Part model, mm, in its own coordinate system. A direction names the side the tool comes from. Coordinates: 2 decimals unless noted, no trailing zeros. Order: outer loops, then holes, each group sorted by start corner. A loop starts at its lowest first (then second) coordinate and runs counter-clockwise, first axis right, second up. Notation, with made-up numbers: M 70.25,73.5 L 128.25,73.5 A24 ccw 128.25,91.5 Z; hole C 50,55.25 d8. An arc over 180 degrees is marked long. Write item = value, one per line. Start each with the question number.
from build123d import *

# Parameters (mm, degrees)
SKETCH1_W           = 10
SKETCH1_H           = 10
BOSS_EXTRUDE1_DEPTH = 10
SKETCH2_R           = 2.5
BOSS_EXTRUDE2_DEPTH = 10
SKETCH3_R           = 2.5
CUT_EXTRUDE1_DEPTH  = 10
SKETCH4_R           = 2.5
CUT_EXTRUDE2_DEPTH  = 10


with BuildPart() as part:
    # Sketch1 → Boss-Extrude1 (new body)
    with BuildSketch(Plane.XY):
        with Locations((5, 5)):
            Rectangle(SKETCH1_W, SKETCH1_H)
    extrude(amount=BOSS_EXTRUDE1_DEPTH)

    # Sketch2 → Boss-Extrude2 (add)
    with BuildSketch(Plane(origin=(0, 10, 0), x_dir=(1, 0, 0), z_dir=(0, 1, 0))):
        with Locations(Location((5, -5, 0), (0, 0, 270))):
            Circle(SKETCH2_R)
    extrude(amount=BOSS_EXTRUDE2_DEPTH)

    # Sketch3 → Cut-Extrude1 (cut)
    with BuildSketch(Plane.XY.offset(10)):
        with Locations((5, 5)):
            Circle(SKETCH3_R)
    extrude(amount=-CUT_EXTRUDE1_DEPTH, mode=Mode.SUBTRACT)

    # Sketch4 → Cut-Extrude2 (cut)
    with BuildSketch(Plane(origin=(10, 0, 0), x_dir=(0, 0, -1), z_dir=(1, 0, 0))):
        with Locations(Location((-5, 5, 0), (0, 0, 90))):
            Circle(SKETCH4_R)
    extrude(amount=-CUT_EXTRUDE2_DEPTH, mode=Mode.SUBTRACT)


solid = part.part
Item 1: Cut at C-C, the plane x = 7. Write the cut outline in (y, z), and give its area (3 significant figures).
Item 2: 3-axis set-ups, long thin cutter, end or side, ignore diameter. For faces 1 (the flat face through (3, 7, 0)), 2 (the cylindrical face through (5.751, 14.93, 7.385)): which of +Z, -Z, +X, -X, +Y, -Y reach the whole face in a straight line?
Item 3: Flat gauge pins, fed straight in: pin 1 (4 mm diameter, centred on x = 5, y = 5, fed in from -Z); pin 2 (4 mm diameter, centred on y = 15.5, z = 2, fed in from -X). Where does each tip first touch, or does it go through?
Item 4: Cut at D-D, the plane x = 8.25. Write the cut outline in (y, z), and give its area (3 significant figures).
Item 5: Wall check: line 1 along Y through (x, z) = (5, 8.25); line 2 along Y through (x, z) = (5, 6.25). Give the ranges that are in metal, low to high. Write a range as [from, to].
Item 6: Cut at B-B, the plane z = 3. Write the cut outline in (x, y), and give its area (3 significant figures).
Item 7: Pull direction Y, two halves, no side cores. Call faces 3 (the flat face through (3, 10, 3)), 4 (the cylindrical face through (6.34, 7.11, 8.09)), 5 (the flat face through (10, 3, 3)): pulls with the +Y half, pulls with the -Y half, needs draft (parallel to the pull), parting line crosses it, or undercut.
Item 8: Cut at A-A, the plane y = 5. Write the cut outline in (x, z), and give its area (3 significant figures).
Filled sheet:
q1.outline = M 0,0 L 3.5,0 L 3.5,3 A2.5 cw 3.5,7 L 3.5,10 L 0,10 Z; M 6.5,0 L 10,0 L 10,3.5 L 20,3.5 L 20,6.5 L 10,6.5 L 10,10 L 6.5,10 L 6.5,7 A2.5 cw 6.5,3 Z
q1.area = 94.4 mm2
q2.face_1 = -Z, +X, -X, +Y, -Y
q2.face_2 = +Y
q3.pin_1 = through
q3.pin_2 = 2.71
q4.outline = M 0,0 L 10,0 L 10,10 L 0,10 Z; hole C 5,5 d5
q4.area = 80.4 mm2
q5.line_1 = [0, 2.5], [7.5, 10]
q5.line_2 = [0, 2.5], [7.5, 20]
q6.outline = M 0,0 L 10,0 L 10,3.5 L 7,3.5 A2.5 cw 3,3.5 L 0,3.5 Z; M 0,6.5 L 3,6.5 A2.5 cw 7,6.5 L 10,6.5 L 10,10 L 6.5,10 L 6.5,20 L 3.5,20 L 3.5,10 L 0,10 Z
q6.area = 94.4 mm2
q7.face_3 = pulls with the +Y half
q7.face_4 = undercut
q7.face_5 = needs draft
q8.outline = M 0,0 L 2.5,0 L 2.5,2.5 L 0,2.5 Z; M 0,7.5 L 2.5,7.5 L 2.5,10 L 0,10 Z; M 7.5,0 L 10,0 L 10,2.5 L 7.5,2.5 Z; M 7.5,7.5 L 10,7.5 L 10,10 L 7.5,10 Z
q8.area = 25.0 mm2
